Can you work these out from the model? Positions are in its coordinate system, mm. Give positions to 0.01 mm unless a question says otherwise; leave off trailing zeros. Loops run counter-clockwise (first coordinate to the right, second up) from the corner with the lowest first, then second, coordinate; pieces in that order, holes last. Notation, with made-up numbers: (5.5, 60.5) - (17.5, 60.5) arc R23 ccw to (17.5, 69.5) - close; hole circle Ø6 at (37, -19). An arc over 180 degrees is marked (long way). Use a Markdown table: item, result. Add a question column.
```python
from build123d import *

# Parameters (mm, degrees)
SKETCH1_W               = 19.05
SKETCH1_H               = 19.05
SKETCH1_W_2             = 15.875
SKETCH1_H_2             = 15.875
BOSS_EXTRUDE1_DEPTH     = 431.8
CUT_EXTRUDE1_REACH      = 434.325
SKETCH2_R               = 3.96875
CUT_EXTRUDE2_DEPTH      = 433.0100592
CUT_EXTRUDE2_DEPTH_BACK = 433.0100592
SKETCH3_R               = 2.38125


with BuildPart() as part:
    # Sketch1 → Boss-Extrude1 (new body)
    with BuildSketch(Plane(origin=(0, 0, 0), x_dir=(1, 0, 0), z_dir=(0, 1, 0))):
        Rectangle(SKETCH1_W, SKETCH1_H)
        Rectangle(SKETCH1_W_2, SKETCH1_H_2, mode=Mode.SUBTRACT)
    extrude(amount=BOSS_EXTRUDE1_DEPTH)

    # Sketch2 → Cut-Extrude1 (cut, up to next)
    with BuildSketch(Plane.XY.offset(9.525), mode=Mode.PRIVATE) as cut_extrude1_sk1:
        with Locations((0, 152.4)):
            Circle(SKETCH2_R)
    cut_extrude1_tool1 = extrude(cut_extrude1_sk1.sketch, amount=-CUT_EXTRUDE1_REACH, mode=Mode.PRIVATE) & part.part
    add(cut_extrude1_tool1.solids().sort_by_distance((0, 152.4, 9.525))[0], mode=Mode.SUBTRACT)

    # Sketch3 → Cut-Extrude2 (cut, two sides: drawn at the far end of the back side and taken through both)
    with BuildSketch(Plane(origin=(0, 0, 0), x_dir=(0, 0, -1), z_dir=(1, 0, 0)).offset(-CUT_EXTRUDE2_DEPTH_BACK)):
        with Locations((0, 12.7)):
            Circle(SKETCH3_R)
        with Locations((0, 63.5)):
            Circle(SKETCH3_R)
        with Locations((0, 241.3)):
            Circle(SKETCH3_R)
        with Locations((0, 368.3)):
            Circle(SKETCH3_R)
        with Locations((0, 419.1)):
            Circle(SKETCH3_R)
    extrude(amount=CUT_EXTRUDE2_DEPTH + CUT_EXTRUDE2_DEPTH_BACK, mode=Mode.SUBTRACT)


solid = part.part
```
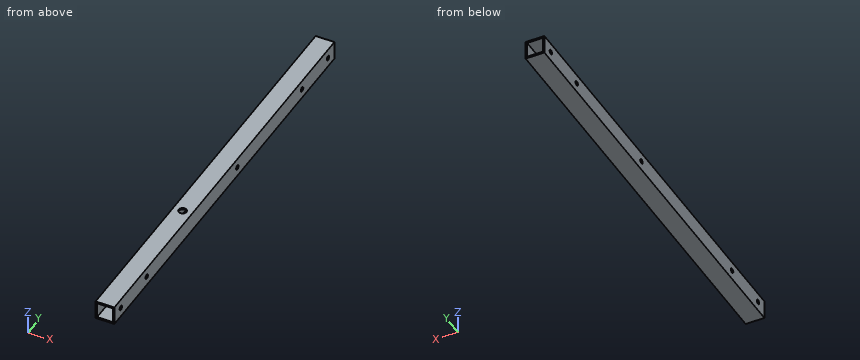
1. Please list where these lines run through material, in increasing order: line 1 along Y through (x, z) = (9.2, 0); line 2 along Z through (x, y) = (-1.5, 22.5) (1 decimal); line 3 along Z through (x, y) = (-9.2, 63.5) (3 decimals). Write a range as [from, to].
2. Will this pin go through, and if not, where does the flat tip stop? P1, Ø7.5, axis at y = 419.1, z = 0, coming from the +X side (3 decimals).
3. Suppose I cut it at C-C (y = 152.4). List the corners of the cut face in (x, z) for me (1 decimal), and give its area (3 significant figures).
4. Suppose I cut it at A-A (x = 0). List the corners of the cut face in (y, z) for me (1 decimal).
5. Suppose I cut it at B-B (y = 278). List the corners of the cut face in (x, z) for me (1 decimal).
Results below:
| question | item | result |
|---|---|---|
| 1 | line 1 | [0, 10.32], [15.08, 61.12], [65.88, 238.92], [243.68, 365.92], [370.68, 416.72], [421.48, 431.8] |
| 1 | line 2 | [-9.5, -7.9], [7.9, 9.5] |
| 1 | line 3 | [-9.525, -2.381], [2.381, 9.525] |
| 2 | P1 | x = 9.525 |
| 3 | outline | (-9.5, -9.5) - (9.5, -9.5) - (9.5, 9.5) - (4, 9.5) - (4, 7.9) - (7.9, 7.9) - (7.9, -7.9) - (-7.9, -7.9) - (-7.9, 7.9) - (-4, 7.9) - (-4, 9.5) - (-9.5, 9.5) - close |
| 3 | area | 98.3 mm² |
| 4 | outline | (0, -9.5) - (431.8, -9.5) - (431.8, -7.9) - (0, -7.9) - close; (0, 7.9) - (148.4, 7.9) - (148.4, 9.5) - (0, 9.5) - close; (156.4, 7.9) - (431.8, 7.9) - (431.8, 9.5) - (156.4, 9.5) - close |
| 5 | outline | (-9.5, -9.5) - (9.5, -9.5) - (9.5, 9.5) - (-9.5, 9.5) - close; hole (-7.9, -7.9) - (7.9, -7.9) - (7.9, 7.9) - (-7.9, 7.9) - close |
